Autodesk Inventor part; units mm, degrees
ref_plane "YZ Plane" through (0, 0, 0) normal (1, 0, 0) x (0, 1, 0)
ref_plane "XZ Plane" through (0, 0, 0) normal (0, 1, 0) x (-1, 0, 0)
ref_plane "XY Plane" through (0, 0, 0) normal (0, 0, 1) x (1, 0, 0)
sketch "Эскиз1" plane through (0, 0, 0) normal (0, 0, 1) x (1, 0, 0)
  line L0 (17.5, -20) -> (-17.5, -20)
  line L1 (-17.5, -20) -> (-17.5, 20)
  line L2 (-17.5, 20) -> (17.5, 20)
  line L3 (17.5, 20) -> (17.5, -20)
  line L4 (17.5, -20) -> (-17.5, 20) construction
  line L5 (-17.5, -20) -> (17.5, 20) construction
  circle A0 centre (0, 0) radius 6.25
  dimension "d0" = 40
  dimension "d1" = 12.5
  dimension "d11" = 35
extrude "Выдавливание1" add sketch "Эскиз1" along normal blind 34
fillet "Сопряжение1" radius 7 4 edges at (-17.5, -20, 17) (-17.5, 20, 17) (17.5, 20, 17) (17.5, -20, 17)
sketch "Эскиз2" plane through (0, 0, 0) normal (0, 0, -1) x (-1, 0, 0)
  line L0 (-10.5, -20) -> (10.5, -20)
  line L1 (10.5, 20) -> (-10.5, 20)
  line L2 (-17.5, 13) -> (-17.5, -13)
  arc A0 (-17.5, -13) -> (-10.5, -20) centre (-10.5, -13) ccw
  arc A1 (10.5, -20) -> (17.5, -13) centre (10.5, -13) ccw
  arc A2 (17.5, 13) -> (10.5, 20) centre (10.5, 13) ccw
  arc A3 (-10.5, 20) -> (-17.5, 13) centre (-10.5, 13) ccw
  line L3 (17.5, -13) -> (17.5, 13)
  line L4 (-12.5, 15) -> (12.5, 15)
  line L5 (12.5, 15) -> (12.5, -15)
  line L6 (12.5, -15) -> (-12.5, -15)
  line L7 (-12.5, -15) -> (-12.5, 15)
  line L8 (-12.5, 15) -> (12.5, -15) construction
  line L9 (12.5, 15) -> (-12.5, -15) construction
  point P0 (0, 0)
  dimension "d12" = 5
  dimension "d13" = 5
extrude "Выдавливание2" cut sketch "Эскиз2" against normal blind 5 contours L4 L5 L6 L7
fillet "Сопряжение3" radius 2 4 edges at (12.5, -15, 2.5) (-12.5, -15, 2.5) (-12.5, 15, 2.5) (12.5, 15, 2.5)
fillet "Сопряжение4" radius 1 8 edges at (-11.9142, 14.4142, 5) (-12.5, 0, 5) (-11.9142, -14.4142, 5) (0, -15, 5) (11.9142, -14.4142, 5) (12.5, 0, 5) (11.9142, 14.4142, 5) (0, 15, 5)
properties part number "платик под двигатель"
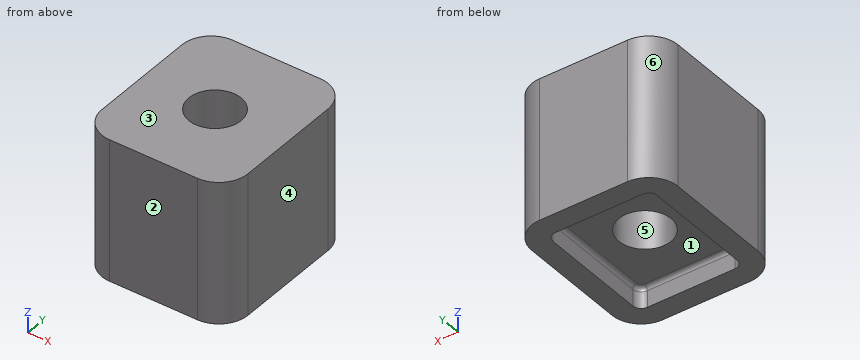
The listing builds one solid part. Answer for the finished solid, in the listing's coordinates (mm). Face numbers are marked on the shaded views. A direction names the side the tool comes from. Give positions to 0.01 mm unless a question says otherwise; leave off trailing zeros. Write each loop counter-clockwise with the first axis right and the second up, starting at its lowest first coordinate (ties: lowest second). Pieces come first, ordered by that corner, then holes. Notation, with made-up numbers: (41.5, 87.5) - (99.5, 87.5) arc R22 cw to (99.5, 108.5) - close; hole circle Ø9 at (38.25, 9.5). An arc over 180 degrees is marked (long way). One line per question, with ' | ' between items. Start each with the question number.
1. Determine the mould class of the marked faces 3, 4, 5 and 6 for opening direction X: +X half, -X half, draft (parallel to the pull), parting line (faces both ways), or undercut.
2. Section B-B, the plane y = 0 is taken. Determine the outline of the cut face in (x, z).
3. Straight lines are drawn through the part: line 1 (Y direction, x = -9, z = 2); line 2 (X direction, y = 0, z = 22.5); line 3 (Y direction, x = 0, z = 16.25). For each, find the intervals that lie inside material, in ascending order.
4. For the marked faces 1 and 2, determine the directions among +Z, -Z, +X, -X, +Y, -Y from which every point of the face is accessible in a straight line to the end or side of a thin tool.
5. Section C-C, the plane y = 7 is taken. Determine the outline of the cut face in (x, z), then the cut area to 3 significant figures.
6. Given P1, Ø11.5, axis at x = 3.5, y = 4, coming from the -Z side; P2, Ø10, axis at x = 0, y = 0, coming from the +Z side; P3, Ø1, axis at y = -14.5, z = 8, coming from the +X side; P4, Ø1, axis at x = -11.5, z = 24.5, coming from the +Y side, each flat-ended and moving along its own axis, determine where each tip first touches the part or whether it passes through.
7. Section D-D, the plane x = -14 is taken. Determine the outline of the cut face in (y, z).
8. Section A-A, the plane x = 0 is taken. Determine the outline of the cut face in (y, z), then the cut area to 3 significant figures.
Result:
1) face 3: draft | face 4: +X half | face 5: undercut | face 6: -X half
2) outline: (-17.5, 0) - (-12.5, 0) - (-12.5, 4) arc R1 cw to (-11.5, 5) - (-6.25, 5) - (-6.25, 34) - (-17.5, 34) - close; (6.25, 5) - (11.5, 5) arc R1 cw to (12.5, 4) - (12.5, 0) - (17.5, 0) - (17.5, 34) - (6.25, 34) - close
3) line 1: y = -20 to -15, 15 to 20 | line 2: x = -17.5 to -6.25, 6.25 to 17.5 | line 3: y = -20 to -6.25, 6.25 to 20
4) face 1: -Z | face 2: +Z, -Z, +X, -X, -Y
5) outline: (-17.5, 0) - (-12.5, 0) - (-12.5, 4) arc R1 cw to (-11.5, 5) - (11.5, 5) arc R1 cw to (12.5, 4) - (12.5, 0) - (17.5, 0) - (17.5, 34) - (-17.5, 34) - close | area: 1,070 mm2
6) P1: stops at z = 5 | P2: passes through | P3: stops at x = 17.43 | P4: stops at y = 19.98
7) outline: (-19.06, 0) - (19.06, 0) - (19.06, 34) - (-19.06, 34) - close
8) outline: (-20, 0) - (-15, 0) - (-15, 4) arc R1 cw to (-14, 5) - (-6.25, 5) - (-6.25, 34) - (-20, 34) - close; (6.25, 5) - (14, 5) arc R1 cw to (15, 4) - (15, 0) - (20, 0) - (20, 34) - (6.25, 34) - close | area: 848 mm2
